Design review of the part shown in the three views and the two pictorial views. Dimensions are in mm from the part's minimum x, y and z. Coordinates: 2 decimals unless noted, no trailing zeros. Loops run counter-clockwise (first coordinate to the right, second up) from the corner with the lowest first, then second, coordinate; pieces in that order, holes last. Notation, with made-up numbers: (64, 64) - (98, 64) arc R27 ccw to (98, 82) - close; hole circle Ø7 at (-33, 50). An arc over 180 degrees is marked (long way). One line per item, written item: value. Start each with the question number.
1. Take a section at A-A, the plane z = 10. State the section outline as (x, y) points.
2. Take a section at C-C, the plane y = 13. State the section outline as (x, z) points, and give its area (3 significant figures).
3. Insertion check: pin 1 (4.5 mm diameter, centred on y = 7, z = 10, fed in from +X); pin 2 (2 mm diameter, centred on y = 13, z = 9.5, fed in from +X). Each pin has a flat end and moves straight along its axis. Give the tip position at first contact, or say it passes through.
4. Take a section at D-D, the plane y = 7.75. State the section outline as (x, z) points, and give its area (3 significant figures).
5. To check wall thickness, follow line 1 (Y direction, x = 11.75, z = 10); line 2 (Z direction, x = 15, y = 7); line 3 (Y direction, x = 15, z = 9.5). State the ranges of each line that lie inside material, in increasing order. Write a range as from..to.
6. Take a section at B-B, the plane x = 10. State the section outline as (y, z) points.
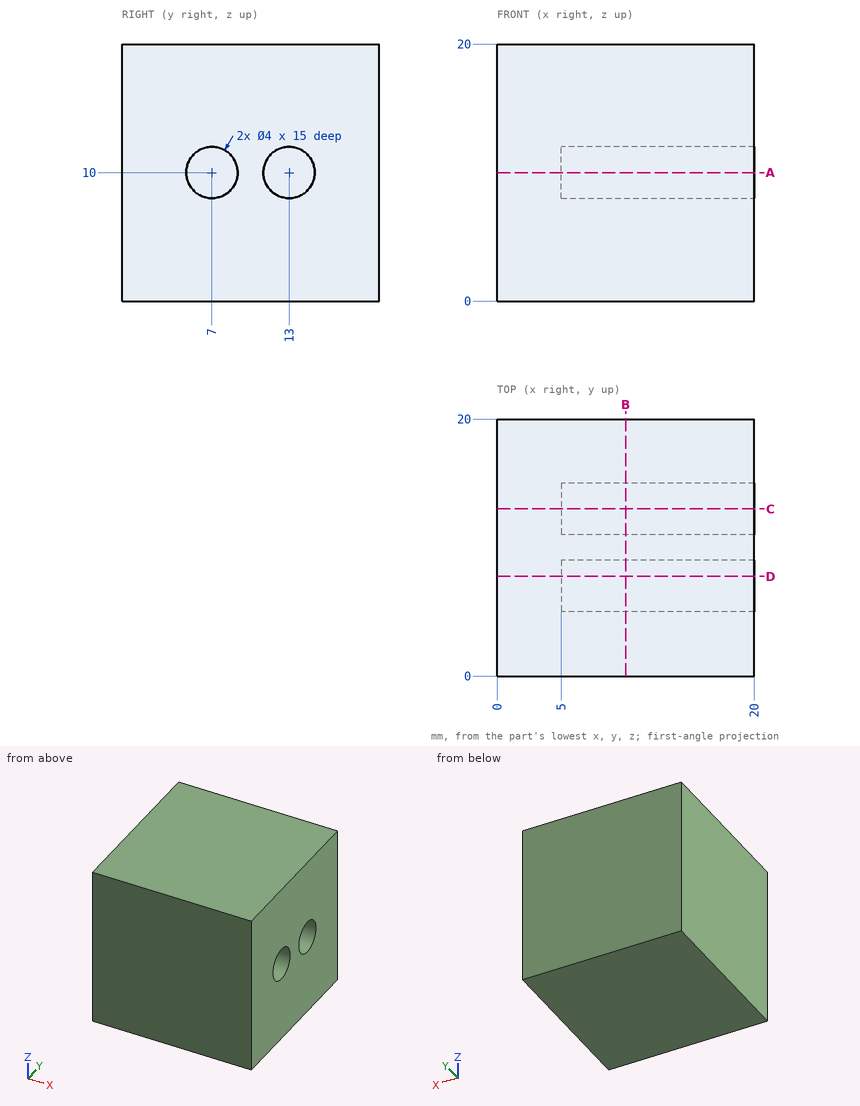
Solutions:
1. outline: (0, 0) - (20, 0) - (20, 5) - (5, 5) - (5, 9) - (20, 9) - (20, 11) - (5, 11) - (5, 15) - (20, 15) - (20, 20) - (0, 20) - close
2. outline: (0, 0) - (20, 0) - (20, 8) - (5, 8) - (5, 12) - (20, 12) - (20, 20) - (0, 20) - close
2. area: 340 mm2
3. pin 1: x = 20
3. pin 2: x = 5
4. outline: (0, 0) - (20, 0) - (20, 8.15) - (5, 8.15) - (5, 11.85) - (20, 11.85) - (20, 20) - (0, 20) - close
4. area: 344 mm2
5. line 1: 0..5, 9..11, 15..20
5. line 2: 0..8, 12..20
5. line 3: 0..5.06, 8.94..11.06, 14.94..20
6. outline: (0, 0) - (20, 0) - (20, 20) - (0, 20) - close; hole circle Ø4 at (7, 10); hole circle Ø4 at (13, 10)
